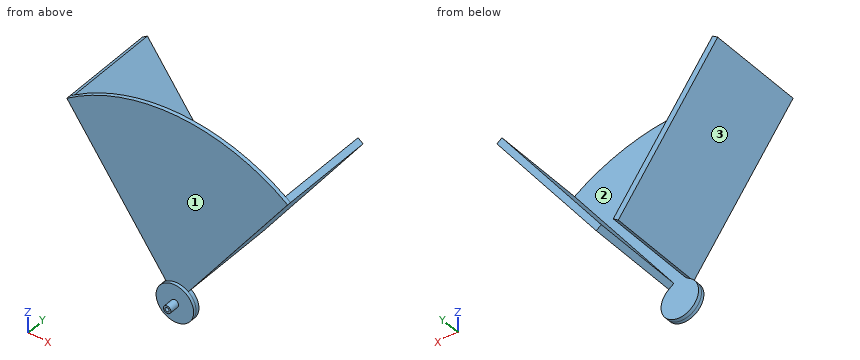
from build123d import *

# Parameters (mm, degrees)
SKETCH1_R           = 6
SKETCH1_R_2         = 3.175
BOSS_EXTRUDE1_DEPTH = 16
SKETCH2_R           = 30
BOSS_EXTRUDE2_DEPTH = 5
BOSS_EXTRUDE3_DEPTH = 6
BOSS_EXTRUDE4_DEPTH = 150


with BuildPart() as part:
    # Sketch1 → Boss-Extrude1 (new body)
    with BuildSketch(Plane(origin=(0, 0, 0), x_dir=(1, 0, 0), z_dir=(0, 1, 0))):
        with Locations(Location((0, 0, 0), (0, 0, 270))):
            Circle(SKETCH1_R)
        with Locations(Location((0, 0, 0), (0, 0, 270))):
            Circle(SKETCH1_R_2, mode=Mode.SUBTRACT)
    extrude(amount=BOSS_EXTRUDE1_DEPTH)

    # Sketch2 → Boss-Extrude2 (add)
    with BuildSketch(Plane(origin=(0, 16, 0), x_dir=(1, 0, 0), z_dir=(0, 1, 0))):
        with Locations(Location((0, 0, 0), (0, 0, 270))):
            Circle(SKETCH2_R)
    extrude(amount=BOSS_EXTRUDE2_DEPTH)

    # Sketch3 → Boss-Extrude3 (add)
    with BuildSketch(Plane(origin=(0, 21, 0), x_dir=(1, 0, 0), z_dir=(0, 1, 0))):
        with BuildLine():
            Line((17.633557569, -24.270509831), (176.335575688, -242.705098312))
            ThreePointArc((176.335575688, -242.705098312), (0, -300), (-176.335575688, -242.705098312))
            Line((-176.335575688, -242.705098312), (-17.633557569, -24.270509831))
            ThreePointArc((-17.633557569, -24.270509831), (0, 30), (17.633557569, -24.270509831))
        make_face()
    extrude(amount=BOSS_EXTRUDE3_DEPTH)

    # Sketch4 → Boss-Extrude4 (add)
    with BuildSketch(Plane(origin=(0, 27, 0), x_dir=(1, 0, 0), z_dir=(0, 1, 0))):
        Polygon((-176.335575688, -242.705098312), (-17.633557569, -24.270509831), (-9.543387625, -30.148362354), (-168.245405744, -248.582950835), align=None)
        Polygon((17.633557569, -24.270509831), (176.335575688, -242.705098312), (168.245405744, -248.582950835), (9.543387625, -30.148362354), align=None)
    extrude(amount=BOSS_EXTRUDE4_DEPTH)


solid = part.part
Read the model definition and answer for the solid it produces. Units are mm, in the model's axes. Face numbers are marked on the shaded views. Coordinates: 2 decimals unless noted, no trailing zeros. Loops run counter-clockwise (first coordinate to the right, second up) from the corner with the lowest first, then second, coordinate; pieces in that order, holes last. Notation, with made-up numbers: (38, 26) -> (83, 26) arc R25 cw to (83, 47) -> close; hole circle Ø9 at (68, -16). An arc over 180 degrees is marked (long way). Write item = value, one per line. Start each with the question number.
1) The part is cut by section C-C, the plane x = -92. Determine the outline of the cut face in (y, z), plus the area to 3 significant figures.
2) The mould has two halves that part along X. Classify the marked faces 1, 2 and 3: pulls with the +X half, pulls with the -X half, needs draft (parallel to the pull), parting line crosses it, or undercut.
3) Given P1, Ø4, axis at y = 151, z = 35.5, coming from the -X side; P2, Ø8, axis at x = 23.5, y = 76.5, coming from the +Z side; P3, Ø5, axis at x = -49, z = 155.5, coming from the +Y side, each flat-ended and moving along its own axis, determine where each tip first touches the part or whether it passes through.
4) The part is cut by section B-B, the plane z = 78. Determine the outline of the cut face in (x, y).
5) The part is cut by section A-A, the plane y = 124.5. Determine the outline of the cut face in (x, z), plus the area to 3 significant figures.
6) The part is cut by section D-D, the plane x = 51. Determine the outline of the cut face in (y, z).
7) Find the intervals of material crossed by L1, parallel to X at y = 12, z = 0 (3 decimals); L2, parallel to Y at x = 8, z = 114; L3, parallel to X at y = 73, z = 81.5, in increasing order. Write a range as from..to.
Result:
q1.outline = (21, 126.63) -> (177, 126.63) -> (177, 143.64) -> (27, 143.64) -> (27, 285.55) -> (21, 285.55) -> close
q1.area = 3,510 mm²
q2.face_1 = needs draft
q2.face_2 = undercut
q2.face_3 = pulls with the -X half
q3.P1 = -27.25
q3.P2 = 54.86
q3.P3 = 27
q4.outline = (-56.67, 21) -> (56.67, 21) -> (56.67, 177) -> (44.31, 177) -> (44.31, 27) -> (-44.31, 27) -> (-44.31, 177) -> (-56.67, 177) -> close
q5.outline = (-176.34, 242.71) -> (-17.63, 24.27) -> (-9.54, 30.15) -> (-168.25, 248.58) -> close; (9.54, 30.15) -> (17.63, 24.27) -> (176.34, 242.71) -> (168.25, 248.58) -> close
q5.area = 5,400 mm²
q6.outline = (21, 70.2) -> (177, 70.2) -> (177, 87.21) -> (27, 87.21) -> (27, 295.63) -> (21, 295.63) -> close
q7.L1 = -6..-3.175, 3.175..6
q7.L2 = 21..27
q7.L3 = -59.21..-46.85, 46.85..59.21
